Autodesk Inventor part; units mm, degrees
ref_plane "Work Plane3-top of part" through (0, 0, 9.525) normal (0, 0, 1) x (1, 0, 0)
ref_plane "Work Plane4 -Assembly Mate Height" through (0, 0, -0.8636) normal (0, 0, 1) x (1, 0, 0)
ref_plane "Work Plane1-between two actuators" through (-29.0322, 0, 0) normal (1, 0, 0) x (0, 1, 0)
ref_plane "Work Plane2-Y position of rear act" through (0, 105.283, 0) normal (0, 1, 0) x (-1, 0, 0)
ref_plane "Work Plane5-Y Position of Front Actuator" through (0, 18.923, 0) normal (0, 1, 0) x (-1, 0, 0)
ref_plane "Work Plane3-top of part" through (0, 0, 9.525) normal (0, 0, 1) x (1, 0, 0)
ref_plane "Work Plane4 -Assembly Mate Height" through (0, 0, -0.8636) normal (0, 0, 1) x (1, 0, 0)
ref_plane "Work Plane6 center of ball tip plane" through (0, 0, -0.2794) normal (0, 0, 1) x (1, 0, 0)
sketch "Sketch5" plane through (0, 0, 0) normal (1, 0, 0) x (0, 1, 0)
  point P0 (0, 0)
sketch "Sketch1" plane through (0, 0, 0) normal (0, 0, 1) x (1, 0, 0)
  line L0 (-38.1, 117.7798) -> (0, 117.7798)
  line L1 (0, 117.7798) -> (0, -2.5908)
  line L2 (-38.1, -2.5908) -> (-38.1, 117.7798)
  line L3 (-38.1, -2.5908) -> (0, -2.5908)
  line L4 (-45.72, 0) -> (7.62, 0)
  line L5 (0, 142.0481) -> (0, -27.8299)
  point P0 (0, 0)
  point P1 (0, -3.5617)
  dimension "d0" = 38.1
  dimension "d55" = 0
  dimension "d135" = 117.7798
  dimension "d136" = 2.5908
extrude "Extrusion1" add sketch "Sketch1" along normal blind 9.525
sketch "Sketch9" plane through (0, 0, 0) normal (0, 0, 1) x (1, 0, 0)
  circle A0 centre (-3.81, 65.7098) radius 1.6002
  circle A1 centre (-3.81, 14.9098) radius 1.6002
  line L0 (0, 117.7798) -> (0, 0)
  line L1 (-6.4922, 0) -> (1.082, 0)
  circle A2 centre (-3.81, 67.31) radius 1.6002
  circle A3 centre (-3.81, 64.1096) radius 1.6002
  line L2 (-5.4102, 67.31) -> (-5.4102, 64.1096)
  line L3 (-2.2098, 67.31) -> (-2.2098, 64.1096)
  line L4 (-3.81, 65.7098) -> (-3.81, 14.9098)
  dimension "d59" = 3.2004
  dimension "d60" = 3.2004
  dimension "d61" = 50.8
  dimension "d62" = 3.81
  dimension "d63" = 14.9098
extrude "Locating Pin features Extrusion7" cut sketch "Sketch9" along normal blind 6.35
sketch "Sketch10" plane through (0, 0, 9.525) normal (0, 0, 1) x (1, 0, 0)
  circle A0 centre (-3.81, 14.9098) radius 1.6002
  circle A1 centre (-3.81, 23.1648) radius 1.5875
  circle A2 centre (-3.81, 73.9648) radius 1.5875
  arc A3 (-2.2098, 67.31) -> (-5.4102, 67.31) centre (-3.81, 67.31) ccw
  arc A4 (-5.4102, 64.1096) -> (-2.2098, 64.1096) centre (-3.81, 64.1096) ccw
  line L0 (-5.4102, 64.1096) -> (-5.4102, 67.31)
  line L1 (-2.2098, 67.31) -> (-2.2098, 64.1096)
  line L2 (-5.4102, 65.7098) -> (-2.2098, 65.7098)
  line L3 (-3.81, 65.7098) -> (-3.81, 14.9098)
  point P0 (0, 0)
  point P1 (-3.81, 48.5648)
  dimension "d67" = 3.175
  dimension "d68" = 3.175
  dimension "d69" = 50.8
  dimension "d282" = 23.1648
  dimension "d295" = 25.4
hole "Mtg Holes Hole2" at (-3.81, 23.1648, 9.525) at (-3.81, 73.9648, 9.525) at (-3.81, 48.5648, 9.525) direction (0, 0, -1) diameter 4.4958 end through all
sketch "Sketch22" plane through (0, 0, 0) normal (0, 0, 1) x (1, 0, 0)
  circle A0 centre (-29.0418, 18.923) radius 2.54 construction
  line L0 (-41.6966, 105.283) -> (6.9494, 105.283) construction
  line L1 (-34.7472, 93.218) -> (-23.3172, 93.218)
  line L2 (-23.3172, 93.218) -> (-23.3172, 81.788)
  line L3 (-23.3172, 81.788) -> (-34.7472, 81.788)
  line L4 (-34.7472, 81.788) -> (-34.7472, 93.218)
  line L5 (-23.3172, 87.503) -> (-34.7472, 87.503) construction
  line L6 (-34.7472, 38.608) -> (-23.3172, 38.608)
  line L7 (-23.3172, 38.608) -> (-23.3172, 27.178)
  line L8 (-23.3172, 27.178) -> (-34.7472, 27.178)
  line L9 (-34.7472, 27.178) -> (-34.7472, 38.608)
  line L10 (-23.3172, 32.893) -> (-34.7472, 32.893) construction
  line L11 (-41.6966, 18.923) -> (6.9494, 18.923)
  line L12 (-29.0322, 111.8616) -> (-29.0322, -18.6436)
  line L13 (-29.0322, 93.218) -> (-29.0322, 81.788) construction
  line L14 (-29.0322, 93.218) -> (-29.0322, 81.788) construction
  line L15 (-29.0322, 38.608) -> (-29.0322, 27.178) construction
  dimension "d149" = 11.43
  dimension "d150" = 11.43
  dimension "d225" = 13.97
  dimension "d226" = 17.78
  dimension "d227" = 0
extrude "Extrusion13" cut sketch "Sketch22" along normal through all contours L1 L12 L3 L4 | L1 L2 L3 L12
sketch "Sketch38" plane through (0, 0, 9.525) normal (0, 0, 1) x (1, 0, 0)
  line L0 (-38.1, -2.5908) -> (-38.1, 117.7798)
  line L1 (0, -2.5908) -> (-38.1, -2.5908)
  line L2 (-38.1, -0.6858) -> (0, -0.6858)
  line L3 (0, -0.6858) -> (0, 12.065)
  line L4 (0, 12.065) -> (-38.1, 12.065)
  line L5 (-38.1, 12.065) -> (-38.1, -0.6858)
  line L6 (-20.1422, -0.6858) -> (0, -0.6858)
  line L7 (0, -0.6858) -> (0, -2.5908)
  line L8 (0, -2.5908) -> (-20.1422, -2.5908)
  line L9 (-20.1422, -2.5908) -> (-20.1422, -0.6858)
  point P0 (0, 0)
  dimension "d302" = 17.9578
  dimension "d303" = 1.905
  dimension "d304" = 12.7508
extrude "Extrusion22" cut sketch "Sketch38" against normal blind 5.6134 contours L0 L4 L3 L2 | L9 L2 L7 L1
sketch "Sketch39" plane through (0, 0, 0) normal (0, 0, 1) x (1, 0, 0)
  line L0 (-38.1, -0.6858) -> (-38.1, 12.065)
  line L1 (-38.1, 12.065) -> (0, 12.065)
  point P0 (0, 0)
  point P1 (-20.955, 5.6896)
  dimension "d307" = 17.145
  dimension "d308" = 6.3754
hole "Hole10" at (-20.955, 5.6896, 0) direction (0, 0, 1) diameter 4.1402 end through all
sketch "Sketch40" plane through (0, 0, 9.525) normal (0, 0, 1) x (1, 0, 0)
  line L0 (-20.1422, -0.6858) -> (-38.1, -0.6858)
  line L1 (-38.1, -2.5908) -> (-38.1, -0.6858)
  line L2 (-20.1422, -2.5908) -> (-20.1422, -0.6858)
  line L3 (-20.1422, -2.5908) -> (-38.1, -2.5908)
  circle A0 centre (-20.955, 5.6896) radius 2.0701
  line L4 (-38.1, -0.6858) -> (-20.1422, -0.6858)
  line L5 (-20.1422, -0.6858) -> (-20.1422, -2.5908)
  line L6 (-20.1422, -2.5908) -> (-38.1, -2.5908)
  line L7 (-38.1, -2.5908) -> (-38.1, -0.6858)
  circle A1 centre (-20.955, 5.6896) radius 9.525
  point P0 (0, 0)
  dimension "d316" = 19.05
extrude "Extrusion23" cut sketch "Sketch40" against normal blind 2.4384 contours L2 L3 A1 L0 | L0 A1 L3 L2 | A1 L3 L1 L0 | A0
sketch "Sketch34" plane through (0, 0, 9.525) normal (0, 0, 1) x (1, 0, 0)
  circle A0 centre (-3.81, 73.9648) radius 2.2479
  circle A1 centre (-3.81, 23.1648) radius 2.2479
  line L0 (0, 117.7798) -> (0, -2.5908)
  line L1 (0, -2.5908) -> (-38.1, -2.5908)
  line L2 (-3.81, 73.9648) -> (-3.81, 23.1648)
  line L3 (-15.4375, 59.5648) -> (-15.4375, 37.5648)
  line L4 (0, 141.8539) -> (0, -26.6649)
  point P0 (0, 0)
  point P1 (-15.4375, 48.5648)
  point P2 (-3.81, 48.5648)
  dimension "d269" = 22
  dimension "d270" = 15.4375
hole "Hole9" at (-15.4375, 59.5648, 9.525) at (-15.4375, 37.5648, 9.525) direction (0, 0, -1) diameter 2.4638 end through all
fillet "Fillet10" radius 2.54 4 edges at (-23.3172, 93.218, 4.7625) (-23.3172, 81.788, 4.7625) (-34.7472, 81.788, 4.7625) (-34.7472, 93.218, 4.7625)
sketch "Sketch24" plane through (0, 0, 0) normal (0, 0, 1) x (1, 0, 0)
  circle A0 centre (-32.8422, 76.708) radius 1.27
  circle A1 centre (-25.2222, 76.708) radius 1.27
  line L0 (-41.6966, 105.283) -> (6.9494, 105.283)
  line L1 (-34.7472, 84.328) -> (-34.7472, 90.678) construction
  line L2 (-34.7472, 87.503) -> (-31.3197, 87.503) construction
  line L3 (-29.0322, 170.9362) -> (-29.0322, -28.4894) construction
  line L4 (-29.0322, 105.283) -> (-29.0322, 142.4468) construction
  dimension "d167" = 2.54
  dimension "d168" = 7.62
  dimension "d236" = 10.795
hole "Hole4" [suppressed]
sketch "Sketch31" plane through (0, 0, 9.525) normal (0, 0, 1) x (1, 0, 0)
  line L0 (-45.72, 105.283) -> (7.62, 105.283)
  line L1 (-29.0322, 141.8539) -> (-29.0322, -26.6649)
  point P0 (0, 0)
  point P1 (-29.0322, 105.283)
hole "Hole6" [suppressed]
sketch "Sketch33" plane through (0, 0, 0) normal (0, 0, -1) x (-1, 0, 0)
  line L0 (-7.62, 105.283) -> (45.72, 105.283)
  line L1 (29.0322, -26.6649) -> (29.0322, 141.8539)
  point P0 (0, 0)
  point P1 (29.0322, 105.283)
hole "Hole8" at (-29.0322, 105.283, 0) direction (0, 0, 1) diameter 13.081 depth 4.5466 counterbore diameter 15.875 counterbore depth 2.54
sketch "Sketch44" plane through (0, 0, 0) normal (0, 0, -1) x (-1, 0, 0)
  circle A0 centre (25.2222, 76.708) radius 1.2319
  circle A1 centre (32.8422, 76.708) radius 1.2319
  line L0 (23.3172, 84.328) -> (23.3172, 90.678)
  arc A2 (25.8572, 93.218) -> (23.3172, 90.678) centre (25.8572, 90.678) ccw
  line L1 (25.8572, 93.218) -> (32.2072, 93.218)
  line L2 (34.7472, 90.678) -> (34.7472, 84.328)
  line L3 (32.2072, 81.788) -> (25.8572, 81.788)
  line L4 (23.3172, 90.678) -> (34.7472, 90.678)
  line L5 (34.7472, 90.678) -> (34.7472, 72.898)
  line L6 (34.7472, 72.898) -> (23.3172, 72.898)
  line L7 (23.3172, 72.898) -> (23.3172, 90.678)
  point P0 (0, 0)
  dimension "d341" = 8.89
extrude "Extrusion24" cut sketch "Sketch44" against normal blind 2.54 contours A0 | A1 | L0 L4 L2 L5 L6 L7
fillet "Fillet27" radius 2.54 2 edges at (-23.3172, 72.898, 1.27) (-34.7472, 72.898, 1.27)
chamfer "Chamfer17" distance 0.635 angle 45 8 edges at (-23.3172, 83.058, 0) (-24.0611, 92.4741, 0) (-29.0322, 93.218, 0) (-34.0033, 92.4741, 0) (-34.7472, 83.058, 0) (-34.0033, 73.6419, 0) (-29.0322, 72.898, 0) (-24.0611, 73.6419, 0)
sketch "Sketch35" plane through (0, 0, 0) normal (0, 0, 1) x (1, 0, 0)
  line L0 (-38.1, 117.7798) -> (0, 117.7798)
  line L1 (0, 117.7798) -> (0, 12.065)
  line L2 (0, 117.7798) -> (-15.875, 117.7798)
  line L3 (-15.875, 117.7798) -> (-15.875, 80.9498)
  line L4 (-15.875, 80.9498) -> (0, 80.9498)
  line L5 (0, 80.9498) -> (0, 117.7798)
  line L6 (-38.1, 12.065) -> (-38.1, 117.7798)
  point P0 (0, 0)
  point P1 (0, 4.3942)
  point P2 (-38.1, -2.5908)
  point P3 (0, 1.8542)
  point P4 (0, -2.5908)
  dimension "d283" = 15.875
  dimension "d284" = 22.225
  dimension "d285" = 36.83
extrude "Extrusion19" cut sketch "Sketch35" along normal blind 25.4
sketch "Sketch37" plane through (0, 0, 9.525) normal (0, 0, 1) x (1, 0, 0)
  circle A0 centre (-3.81, 48.5648) radius 2.2479
  circle A1 centre (-3.81, 73.9648) radius 2.2479
  circle A2 centre (-3.81, 23.1648) radius 2.2479
  circle A3 centre (-3.81, 73.9648) radius 4.1275
  circle A4 centre (-3.81, 48.5648) radius 4.1275
  circle A5 centre (-3.81, 23.1648) radius 4.1275
  line L0 (-3.81, 78.0923) -> (0.3175, 78.0923)
  line L1 (0.3175, 78.0923) -> (0.3175, 69.8373)
  line L2 (0.3175, 69.8373) -> (-3.81, 69.8373)
  line L3 (-3.81, 69.8373) -> (-3.81, 78.0923)
  line L4 (-3.81, 52.6923) -> (0.3175, 52.6923)
  line L5 (0.3175, 52.6923) -> (0.3175, 44.4373)
  line L6 (0.3175, 44.4373) -> (-3.81, 44.4373)
  line L7 (-3.81, 44.4373) -> (-3.81, 52.6923)
  line L8 (-3.81, 27.2923) -> (0.3175, 27.2923)
  line L9 (0.3175, 27.2923) -> (0.3175, 19.0373)
  line L10 (0.3175, 19.0373) -> (-3.81, 19.0373)
  line L11 (-3.81, 19.0373) -> (-3.81, 27.2923)
  point P0 (0, 0)
  dimension "d298" = 8.255
extrude "Extrusion21" cut sketch "Sketch37" against normal blind 5.715 contours A0 L7 | A0 L7 A4 | A0 L7 A4 | L4 L5 A4 | A4 L5 L6 | A1 L3 | A1 L3 A3 | A1 L3 A3 | L0 L1 A3 | A3 L1 L2 | A2 L11 | A2 L11 A5 | A2 L11 A5 | L8 L9 A5 | A5 L9 L10 picked at (-2.5903, 49.1767) picked at (-3.3428, 74.5506) picked at (-3.0093, 23.7506)
chamfer "Chamfer12" distance 0.635 angle 45 1 edges at (-29.0322, 97.3455, 0)
fillet "Fillet20" radius 6.35 1 edges at (-15.875, 80.9498, 4.7625)
fillet "Fillet21" radius 3.175 2 edges at (-15.875, 117.7798, 4.7625) (-38.1, 117.7798, 4.7625)
fillet "Fillet23" [suppressed]
chamfer "Chamfer13" distance 1.905 angle 45 2 edges at (-20.1422, -1.6383, 7.0866) (-38.1, -1.6383, 7.0866)
chamfer "Chamfer14" distance 6.985 angle 45 1 edges at (0, -2.5908, 1.9558)
fillet "Fillet24" radius 1.27 2 edges at (0, 4.3942, 1.9558) (-6.985, -2.5908, 1.9558)
chamfer "Chamfer15" distance 0.635 angle 45 1 edges at (-20.955, 15.2146, 9.525)
fillet "Fillet25" radius 1.27 2 edges at (-13.8783, 12.065, 7.9883) (-28.0317, 12.065, 7.9883)
chamfer "Chamfer16" distance 3.175 angle 45 4 edges at (0, 15.5512, 9.525) (0, 35.8648, 9.525) (0, 61.2648, 9.525) (0, 79.5211, 9.525)
fillet "Fillet26" radius 1.27 8 edges at (0, 12.065, 5.1308) (0, 19.0373, 5.08) (0, 27.2923, 5.08) (0, 44.4373, 5.08) (0, 52.6923, 5.08) (0, 69.8373, 5.08) (0, 78.0923, 5.08) (0, 80.9498, 3.175)
sketch "Sketch41" plane through (0, 0, 9.525) normal (0, 0, 1) x (1, 0, 0)
  circle A0 centre (-15.4375, 37.5648) radius 1.2319
  circle A1 centre (-15.4375, 59.5648) radius 1.2319
  line L0 (-32.2072, 93.218) -> (-25.8572, 93.218)
  line L1 (-15.4375, 59.5648) -> (-15.4375, 37.5648) construction
  point P0 (0, 0)
  point P1 (-15.4375, 48.5648)
hole "Hole11" at (-15.4375, 48.5648, 9.525) direction (0, 0, -1) diameter 11.43 depth 3.81
fillet "Fillet28" radius 1.27 1 edges at (-38.1, 12.065, 6.7183)
properties part number "J002875" material "ALUMINUM, 6061-T651"
Read the model definition and answer for the solid it produces. Units are mm, in the model's axes. A direction names the side the tool comes from. Give positions to 0.01 mm unless a question says otherwise; leave off trailing zeros. Write each loop counter-clockwise with the first axis right and the second up, starting at its lowest first coordinate (ties: lowest second). Pieces come first, ordered by that corner, then holes. Notation, with made-up numbers: (32, -13.5) - (49, -13.5) arc R30 ccw to (49, 19.5) - close; hole circle Ø3 at (43, -12). An arc over 180 degrees is marked (long way). Use CSV: the item, a comma, the result in double quotes. Start each with the question number.
Item 1: The part is cut by section B-B, the plane y = 23.5. Give the vertices of the cut face in (x, z) (3 decimals), and give its area (3 significant figures).
Item 2: Flat-ended cylindrical pins translate along their axes: P1, Ø18.5, axis at x = -29.03, y = 105.28, coming from the -Z side; P2, Ø5, axis at x = -4, z = 3, coming from the -Y side; P3, Ø10.5, axis at x = -15.44, y = 48.56, coming from the +Z side (3 decimals); P4, Ø6.5, axis at x = -2.5, y = 23.5, coming from the +Z side. Find the tip coordinate at first contact, or state that the pin passes through.
Item 3: The part is cut by section A-A, the plane y = 48. Give the vertices of the cut face in (x, z) (3 decimals).
Item 4: The part is cut by section C-C, the plane y = 95. Give the vertices of the cut face in (x, z) (3 decimals).
Item 5: The mould has two halves that part along Y. Classify faces 1 (the flat face through (-3.449, 0.945, 1.928)), 2 (the cylindrical face through (-37.15, 116.87, 4.83)), 3 (the flat face through (-2.21, 66, 3)): pulls with the +Y half, pulls with the -Y half, needs draft (parallel to the pull), parting line crosses it, or undercut.
Item 6: For faces 4 (the cylindrical face through (-34.02, 82.55, 6.08)), 5 (the cylindrical face through (-7.937, 74.056, 6.708)), 6 (the conical face through (-24, 92.6, 0.5)), determine the directions among +Z, -Z, +X, -X, +Y, -Y from which every point of the face is accessible in a straight line to the end or side of a thin tool.
Item 7: Consider line 1 (Y direction, x = -3, z = 8.25) (3 decimals); line 2 (Y direction, x = -28, z = 4.75) (3 decimals); line 3 (X direction, y = 90, z = 5.5) (3 decimals). Determine where each line is inside the solid, lowest interval first.
Taken from the geometry:
1,outline,"(-38.1, 0) - (-6.033, 0) - (-6.033, 3.81) - (-7.924, 3.81) - (-7.924, 9.525) - (-38.1, 9.525) - close; (-1.587, 0) - (0, 0) - (0, 3.81) - (-1.587, 3.81) - close"
1,area,"301 mm2"
2,P1,"z = 0"
2,P2,"y = -2.11"
2,P3,"z = 5.715"
2,P4,"z = 3.81"
3,outline,"(-38.1, 0) - (-5.986, 0) - (-5.986, 3.81) - (-7.899, 3.81) - (-7.899, 9.525) - (-9.75, 9.525) - (-9.75, 5.715) - (-21.125, 5.715) - (-21.125, 9.525) - (-38.1, 9.525) - close; (-1.634, 0) - (0, 0) - (0, 3.81) - (-1.634, 3.81) - close"
4,outline,"(-38.1, 0) - (-15.875, 0) - (-15.875, 9.525) - (-38.1, 9.525) - close"
5,face 1,"pulls with the -Y half"
5,face 2,"pulls with the +Y half"
5,face 3,"undercut"
6,face 4,"+Z, -Z"
6,face 5,"+Z, +X"
6,face 6,"-Z"
7,line 1,"12.065 to 19.037, 27.292 to 44.437, 52.692 to 69.837, 78.092 to 80.95"
7,line 2,"-2.591 to -0.686, 12.065 to 81.788, 93.218 to 117.78"
7,line 3,"-38.1 to -34.747, -23.317 to -15.875"
